from build123d import *

# Parameters (mm, degrees)
F1_DEPTH = 2.54
F2_DEPTH = 5.461


with BuildPart() as f1:
    # F0 (on Top) → F1 (new body)
    with BuildSketch(Plane.XY):
        with BuildLine():
            Line((0, 0), (0, 1.5875))
            ThreePointArc((0, 1.5875), (-1.122532, 1.122532), (-1.5875, 0))
            Line((-1.5875, 0), (0, 0))
        make_face()
        with BuildLine():
            ThreePointArc((-32.279158, 0), (-32.744126, 1.122532), (-33.866658, 1.5875))
            Line((-33.866658, 1.5875), (-33.866658, 0))
            Line((-33.866658, 0), (-32.279158, 0))
        make_face()
        with BuildLine():
            ThreePointArc((-1.5875, 0), (-1.122532, 1.122532), (0, 1.5875))
            Line((0, 1.5875), (0, 12.7))
            Line((0, 12.7), (-33.866658, 12.7))
            Line((-33.866658, 12.7), (-33.866658, 9.68375))
            Line((-33.866658, 9.68375), (-33.866658, 7.14375))
            Line((-33.866658, 7.14375), (-33.866658, 1.5875))
            ThreePointArc((-33.866658, 1.5875), (-32.744126, 1.122532), (-32.279158, 0))
            Line((-32.279158, 0), (-25.961585, 0))
            Line((-25.961585, 0), (-23.421585, 0))
            Line((-23.421585, 0), (-16.473984, 0))
            Line((-16.473984, 0), (-13.933984, 0))
            Line((-13.933984, 0), (-1.5875, 0))
        make_face()
        Polygon((-30.256754, 10.16), (-27.716754, 10.16), (-25.176754, 10.16), (-20.635653, 10.16), (-18.095653, 10.16), (-15.555653, 10.16), (-13.015653, 10.16), (-10.475653, 10.16), (-7.664961, 10.16), (-2.54, 10.16), (-2.54, 5.528615), (-2.54, 2.988615), (-2.54, 2.54), (-4.583576, 2.54), (-7.123576, 2.54), (-9.663576, 2.54), (-12.203576, 2.54), (-16.744676, 2.54), (-19.284676, 2.54), (-21.824676, 2.54), (-24.364676, 2.54), (-31.326658, 2.54), (-31.326658, 8.831487), (-31.326658, 10.16), align=None, mode=Mode.SUBTRACT)
        Polygon((-25.176754, 10.16), (-27.716754, 10.16), (-19.284676, 2.54), (-16.744676, 2.54), align=None)
        Polygon((-21.824676, 2.54), (-30.256754, 10.16), (-31.326658, 10.16), (-31.326658, 8.831487), (-24.364676, 2.54), align=None)
        Polygon((-18.095653, 10.16), (-20.635653, 10.16), (-12.203576, 2.54), (-9.663576, 2.54), align=None)
        Polygon((-13.015653, 10.16), (-15.555653, 10.16), (-7.123576, 2.54), (-4.583576, 2.54), align=None)
        Polygon((-7.664961, 10.16), (-10.475653, 10.16), (-2.54, 2.988615), (-2.54, 5.528615), align=None)
    extrude(amount=F1_DEPTH)

    # F0 (on Top) → F2 (join)
    with BuildSketch(Plane.XY):
        with BuildLine():
            Line((-33.866658, 0), (-33.866658, 1.5875))
            ThreePointArc((-33.866658, 1.5875), (-34.98919, -1.122532), (-32.279158, 0))
            Line((-32.279158, 0), (-33.866658, 0))
        make_face()
        with BuildLine():
            ThreePointArc((1.5875, 0), (1.122532, 1.122532), (0, 1.5875))
            Line((0, 1.5875), (0, 0))
            Line((0, 0), (-1.5875, 0))
            ThreePointArc((-1.5875, 0), (0, -1.5875), (1.5875, 0))
        make_face()
        with BuildLine():
            ThreePointArc((-32.279158, 0), (-32.744126, 1.122532), (-33.866658, 1.5875))
            Line((-33.866658, 1.5875), (-33.866658, 0))
            Line((-33.866658, 0), (-32.279158, 0))
        make_face()
        with BuildLine():
            Line((0, 0), (0, 1.5875))
            ThreePointArc((0, 1.5875), (-1.122532, 1.122532), (-1.5875, 0))
            Line((-1.5875, 0), (0, 0))
        make_face()
    extrude(amount=F2_DEPTH)


solid = f1.part
Could you check a few things on this model? Use its own coordinates, in mm. A direction names the side the tool comes from. Give positions to 0.01 mm unless a question says otherwise; leave off trailing zeros. Order: outer loops, then holes, each group sorted by start corner. A loop starts at its lowest first (then second) coordinate and runs counter-clockwise, first axis right, second up.
1. Suppose I cut it at D-D (x = -23.5). Write out the boundary of the cut face in (y, z).
Answers below:
outline: (0, 0) - (4.05, 0) - (4.05, 2.54) - (0, 2.54) - close; (6.35, 0) - (8.64, 0) - (8.64, 2.54) - (6.35, 2.54) - close; (10.16, 0) - (12.7, 0) - (12.7, 2.54) - (10.16, 2.54) - close
2. I need wall thicknesses on L1, parallel to Y at x = -7, z = 2.1; L2, parallel to Y at x = -5.5, z = 1.5; L3, parallel to Z at x = -10, y = 2.75. Which ranges of each line are inside material? Lowest first, please.
Answers below:
L1: y = 0 to 4.72, 7.02 to 9.56, 10.16 to 12.7
L2: y = 0 to 3.37, 5.66 to 8.2, 10.16 to 12.7
L3: z = 0 to 2.54
3. Suppose I cut it at C-C (z = 4.7). Write out the boundary of the cut face in (x, y) (1 decimal).
Answers below:
outline: circle Ø3.2 at (-33.9, 0); circle Ø3.2 at (0, 0)
4. Suppose I cut it at A-A (z = 1.3). State how many separate pieces and enclosed holes the cut face has, plus the area to 3 significant figures.
Answers below:
separate pieces: 1
enclosed holes: 6
area: 316 mm2
5. Suppose I cut it at B-B (x = -6). Write out the boundary of the cut face in (y, z), plus the area to 3 significant figures.
Answers below:
outline: (0, 0) - (3.82, 0) - (3.82, 2.54) - (0, 2.54) - close; (6.12, 0) - (8.66, 0) - (8.66, 2.54) - (6.12, 2.54) - close; (10.16, 0) - (12.7, 0) - (12.7, 2.54) - (10.16, 2.54) - close
area: 22.6 mm2
6. Which directions (+Z, -Z, +X, -X, +Y, -Y) give clear straight access to the entire face, cutting with the end or side of a thin tool? Please do faces 1 (the flat face through (0, 7, 1)), 2 (the flat face through (-33.867, 7, 1)), 3 (the flat face through (-17, 0, 1)), 4 (the flat face through (-13.821, 6.297, 1.252)).
Answers below:
face 1: +Z, -Z, +X, +Y
face 2: +Z, -Z, -X, +Y
face 3: +Z, -Z, -Y
face 4: +Z, -Z
7. For pin 1 (2 mm diameter, centred on x = -23, z = 1, fed in from -Y); pin 2 (2 mm diameter, centred on y = 7, z = 1.5, fed in from +X); pin 3 (8 mm diameter, centred on x = -30, y = 6, fed in from +Z), each with a flat end and sliding along its axis, tell me the tip position at first contact or that it passes through.
Answers below:
pin 1: stops at y = 0
pin 2: stops at x = 0
pin 3: stops at z = 2.54
